Part model, mm, in its own coordinate system. A direction names the side the tool comes from. Round coordinates to 2 decimals unless told otherwise and drop trailing zeros. Order: outer loops, then holes, each group sorted by start corner. A loop starts at its lowest first (then second) coordinate and runs counter-clockwise, first axis right, second up. Notation, with made-up numbers: (62, 18) -> (118, 18) arc R28 cw to (118, 46) -> close; hole circle Ø6 at (64.5, -33). An arc over 180 degrees is marked (long way). Answer as a JSON object with one key per item and string values. Group by question number.
```python
from build123d import *

# Parameters (mm, degrees)
SKETCH1_R                    = 150
BOSS_EXTRUDE1_DEPTH          = 75
CHAMFER1_SIZE                = 10
BOSS_EXTRUDE3_START          = -75
BOSS_EXTRUDE3_DEPTH          = 10
CHAMFER2_SIZE                = 7
BOSS_EXTRUDE4_DEPTH          = 10
SKETCH4_R                    = 4
CUT_EXTRUDE1_DEPTH           = 258.376062501
CIRPATTERN1_COUNT            = 4
CIRPATTERN1_COPY_1_DEPTH     = 10
CIRPATTERN1_COPY_2_DEPTH     = 10
CIRPATTERN1_COPY_3_DEPTH     = 10
CIRPATTERN1_COPY_4_SKETCH_R  = 4
CIRPATTERN1_COPY_4_DEPTH     = 258.376062501
CIRPATTERN1_COPY_5_SKETCH_R  = 4
CIRPATTERN1_COPY_5_DEPTH     = 258.376062501
CIRPATTERN1_COPY_6_SKETCH_R  = 4
CIRPATTERN1_COPY_6_DEPTH     = 258.376062501
CHAMFER2_OF_CIRPATTERN1_SIZE = 7
CUT_EXTRUDE2_START           = -60
CUT_EXTRUDE2_DEPTH           = 60
CIRPATTERN2_COUNT            = 4
SKETCH7_R                    = 110
BOSS_EXTRUDE5_DEPTH          = 9
BOSS_EXTRUDE5_TAPER          = 45
SKETCH8_R                    = 10
BOSS_EXTRUDE6_DEPTH          = 20


with BuildPart() as part:
    # Sketch1 → Boss-Extrude1 (new body)
    with BuildSketch(Plane(origin=(0, 0, 0), x_dir=(1, 0, 0), z_dir=(0, 1, 0))):
        with Locations(Location((0, 0, 0), (0, 0, 270))):
            Circle(SKETCH1_R)
    extrude(amount=BOSS_EXTRUDE1_DEPTH)

    # Chamfer1
    chamfer1_edges = [part.edges().sort_by_distance(p)[0] for p in [
        (0, 75, -150),
    ]]
    chamfer(chamfer1_edges, length=CHAMFER1_SIZE)

    # Sketch2 → Boss-Extrude3 (add)
    with BuildSketch(Plane(origin=(0, 75, 0), x_dir=(1, 0, 0), z_dir=(0, 1, 0)).offset(BOSS_EXTRUDE3_START)):
        with BuildLine():
            Line((-195.236875483, 37.5), (-195.236875483, -37.5))
            Line((-195.236875483, -37.5), (-145.236875483, -37.5))
            ThreePointArc((-145.236875483, -37.5), (-150, 0), (-145.236875483, 37.5))
            Line((-145.236875483, 37.5), (-195.236875483, 37.5))
        make_face()
    boss_extrude3 = extrude(amount=BOSS_EXTRUDE3_DEPTH)

    # Chamfer2
    chamfer2_edges = [part.edges().sort_by_distance(p)[0] for p in [
        (-195.236875483, 5, -37.5),
        (-195.236875483, 5, 37.5),
    ]]
    chamfer(chamfer2_edges, length=CHAMFER2_SIZE)

    # Sketch3 → Boss-Extrude4 (add)
    with BuildSketch(Plane.XY.offset(37.5)):
        Polygon((-144.19716267, 65), (-170.556875483, 65), (-188.236875483, 10), (-188.236875483, 0), (-145.236875483, 0), align=None)
    boss_extrude4 = extrude(amount=-BOSS_EXTRUDE4_DEPTH)

    # Sketch4 → Cut-Extrude1 (cut, through all)
    with BuildSketch(Plane(origin=(0, 75, 0), x_dir=(1, 0, 0), z_dir=(0, 1, 0))):
        with Locations(Location((-172.618437741, -13.75, 0), (0, 0, 270))):
            Circle(SKETCH4_R)
    cut_extrude1 = extrude(amount=-CUT_EXTRUDE1_DEPTH, mode=Mode.SUBTRACT)

    # Mirror3: Boss-Extrude4, Cut-Extrude1 across plane
    add(boss_extrude4.mirror(Plane.XY))
    add(cut_extrude1.mirror(Plane.XY), mode=Mode.SUBTRACT)

    # CirPattern1: Boss-Extrude3, Boss-Extrude4, Cut-Extrude1 ×4 about axis
    cirpattern1_axis = Axis((0, 0, 0), (0, 1, 0))
    add([boss_extrude3.rotate(cirpattern1_axis, i * 360 / CIRPATTERN1_COUNT) for i in range(1, CIRPATTERN1_COUNT)])
    add([boss_extrude4.rotate(cirpattern1_axis, i * 360 / CIRPATTERN1_COUNT) for i in range(1, CIRPATTERN1_COUNT)])
    add([cut_extrude1.rotate(cirpattern1_axis, i * 360 / CIRPATTERN1_COUNT) for i in range(1, CIRPATTERN1_COUNT)], mode=Mode.SUBTRACT)

    # CirPattern1 copy 1 sketch → CirPattern1 copy 1 (add)
    with BuildSketch(Plane(origin=(-37.5, 0, 0), x_dir=(0, 0, -1), z_dir=(-1, 0, 0))):
        Polygon((-144.19716267, -65), (-170.556875483, -65), (-188.236875483, -10), (-188.236875483, 0), (-145.236875483, 0), align=None)
    extrude(amount=-CIRPATTERN1_COPY_1_DEPTH)

    # CirPattern1 copy 2 sketch → CirPattern1 copy 2 (add)
    with BuildSketch(Plane(origin=(0, 0, 37.5), x_dir=(-1, 0, 0), z_dir=(0, 0, 1))):
        Polygon((-144.19716267, -65), (-170.556875483, -65), (-188.236875483, -10), (-188.236875483, 0), (-145.236875483, 0), align=None)
    extrude(amount=-CIRPATTERN1_COPY_2_DEPTH)

    # CirPattern1 copy 3 sketch → CirPattern1 copy 3 (add)
    with BuildSketch(Plane(origin=(37.5, 0, 0), x_dir=(0, 0, 1), z_dir=(1, 0, 0))):
        Polygon((-144.19716267, -65), (-170.556875483, -65), (-188.236875483, -10), (-188.236875483, 0), (-145.236875483, 0), align=None)
    extrude(amount=-CIRPATTERN1_COPY_3_DEPTH)

    # CirPattern1 copy 4 sketch → CirPattern1 copy 4 (cut, through all)
    with BuildSketch(Plane(origin=(0, 75, 0), x_dir=(0, 0, -1), z_dir=(0, 1, 0))):
        with Locations((-172.618437741, 13.75)):
            Circle(CIRPATTERN1_COPY_4_SKETCH_R)
    extrude(amount=-CIRPATTERN1_COPY_4_DEPTH, mode=Mode.SUBTRACT)

    # CirPattern1 copy 5 sketch → CirPattern1 copy 5 (cut, through all)
    with BuildSketch(Plane(origin=(0, 75, 0), x_dir=(-1, 0, 0), z_dir=(0, 1, 0))):
        with Locations((-172.618437741, 13.75)):
            Circle(CIRPATTERN1_COPY_5_SKETCH_R)
    extrude(amount=-CIRPATTERN1_COPY_5_DEPTH, mode=Mode.SUBTRACT)

    # CirPattern1 copy 6 sketch → CirPattern1 copy 6 (cut, through all)
    with BuildSketch(Plane.ZX.offset(75)):
        with Locations((-172.618437741, 13.75)):
            Circle(CIRPATTERN1_COPY_6_SKETCH_R)
    extrude(amount=-CIRPATTERN1_COPY_6_DEPTH, mode=Mode.SUBTRACT)

    # Chamfer2 of CirPattern1
    chamfer2_of_cirpattern1_edges = [part.edges().sort_by_distance(p)[0] for p in [
        (-37.5, 5, 195.236875483),
        (37.5, 5, 195.236875483),
        (195.236875483, 5, 37.5),
        (195.236875483, 5, -37.5),
        (37.5, 5, -195.236875483),
        (-37.5, 5, -195.236875483),
    ]]
    chamfer(chamfer2_of_cirpattern1_edges, length=CHAMFER2_OF_CIRPATTERN1_SIZE)

    # Sketch6 → Cut-Extrude2 (cut)
    with BuildSketch(Plane(origin=(0, 75, 0), x_dir=(1, 0, 0), z_dir=(0, 1, 0)).offset(CUT_EXTRUDE2_START)):
        with BuildLine():
            Line((-112.583302492, -65), (-129.903810568, -75))
            ThreePointArc((-129.903810568, -75), (-106.066017178, -106.066017178), (-75, -129.903810568))
            Line((-75, -129.903810568), (-65, -112.583302492))
            ThreePointArc((-65, -112.583302492), (-91.923881554, -91.923881554), (-112.583302492, -65))
        make_face()
    cut_extrude2 = extrude(amount=CUT_EXTRUDE2_DEPTH, mode=Mode.SUBTRACT)

    # CirPattern2: Cut-Extrude2 ×4 about axis
    cirpattern2_axis = Axis((0, 75, 0), (0, 1, 0))
    for i in range(1, CIRPATTERN2_COUNT):
        add(cut_extrude2.rotate(cirpattern2_axis, i * 360 / CIRPATTERN2_COUNT), mode=Mode.SUBTRACT)

    # Sketch7 → Boss-Extrude5 (add)
    with BuildSketch(Plane(origin=(0, 75, 0), x_dir=(1, 0, 0), z_dir=(0, 1, 0))):
        Circle(SKETCH7_R)
    extrude(amount=BOSS_EXTRUDE5_DEPTH, taper=BOSS_EXTRUDE5_TAPER)

    # Sketch8 → Boss-Extrude6 (add)
    with BuildSketch(Plane(origin=(0, 84, 0), x_dir=(1, 0, 0), z_dir=(0, 1, 0))):
        with Locations(Location((0, 0, 0), (0, 0, 270))):
            Circle(SKETCH8_R)
    extrude(amount=BOSS_EXTRUDE6_DEPTH)


solid = part.part
```
Q1. Two-plate mould, pull along X, no slides. Class faces 1 (the cylindrical face through (0, 37, -150)), 2 (the flat face through (-70.07, 44.58, 121.365)), 3 (the cylindrical face through (91.586, 44.58, -92.26)), 4 (the flat face through (37.5, 32, 162)): +X half, -X half, draft (parallel to the pull), parting line (faces both ways), or undercut.
Q2. Which spindle directions (+Z, -Z, +X, -X, +Y, -Y) get a long thin tool onto all of the face, cutting with end or side? Do faces 5 (the flat face through (163, 37, 27.5)), 6 (the flat face through (-37.5, 32, 162)), 7 (the flat face through (121.365, 44.58, 70.07)). Say none if no direction does.
Q3. Drop flat-ended pins along their axis: pin 1 Ø13 at (x, y) = (-160.5, 16.5) entering from -Z; pin 2 Ø5 at (x, y) = (90, 50.5) entering from -Z; pin 3 Ø4 at (y, z) = (34, 95) entering from +X (3 decimals). Give the stop position or say it passes through.
Q4. Wall check: line 1 (Z direction, x = 13, y = 6); line 2 (Z direction, x = -13.75, y = 7.5). Give the ranges that are in metal, low to high. Write a range as [from, to].
Q5. Band-saw the part on A-A (x = 0). List the corners of the cut face in (y, z).
Completed:
{
 "1": {"face 1": "undercut", "face 2": "-X half", "face 3": "undercut", "face 4": "+X half"},
 "2": {"face 5": "+X, +Y", "face 6": "+Z, -X, +Y, -Y", "face 7": "+Z, +Y"},
 "3": {"pin 1": "z = -37.5", "pin 2": "z = -96.14", "pin 3": "x = 90.835"},
 "4": {"line 1": "[-195.24, -176.55], [-168.69, 168.69], [176.55, 195.24]", "line 2": "[-195.24, -176.62], [-168.62, 168.62], [176.62, 195.24]"},
 "5": {"outline": "(0, -195.24) -> (10, -195.24) -> (10, -150) -> (65, -150) -> (75, -140) -> (75, -110) -> (84, -101) -> (84, -10) -> (104, -10) -> (104, 10) -> (84, 10) -> (84, 101) -> (75, 110) -> (75, 140) -> (65, 150) -> (10, 150) -> (10, 195.24) -> (0, 195.24) -> close"}
}
